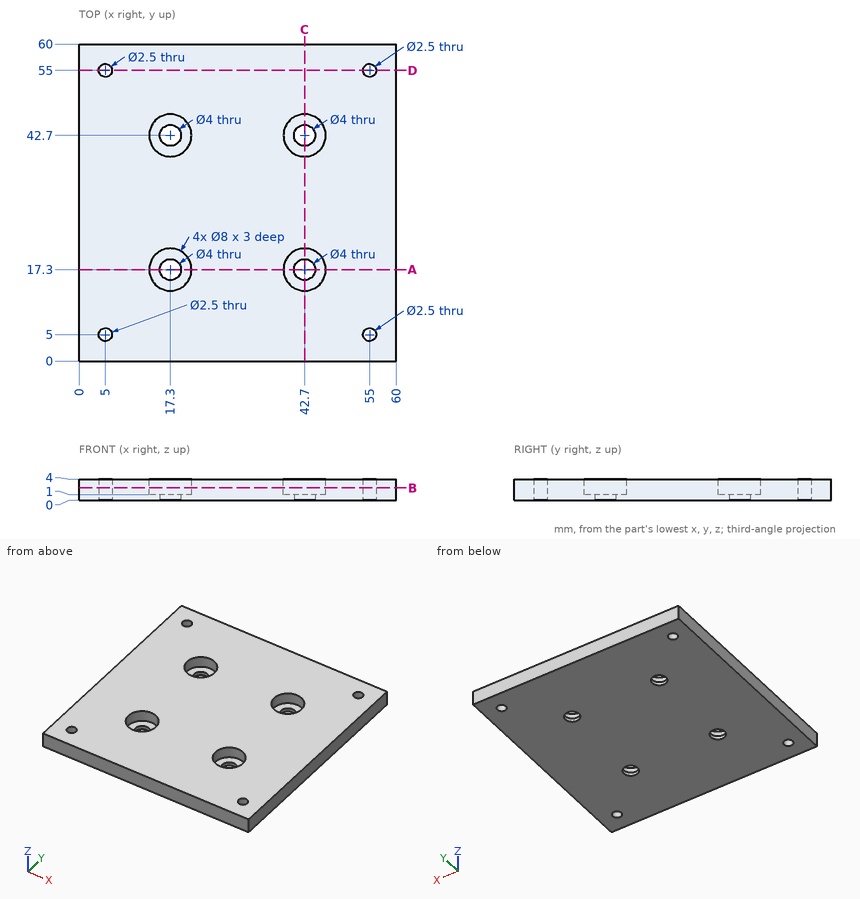
Geometry: see drawing. Coordinates: mm, zero at the bounding-box minimum. Coordinates: 2 decimals unless noted, no trailing zeros. Order: outer loops, then holes, each group sorted by start corner. A loop starts at its lowest first (then second) coordinate and runs counter-clockwise, first axis right, second up. Notation, with made-up numbers: M 59.25,-26 L 98.25,-26 A14 ccw 98.25,-3 Z; hole C 23.5,57 d2. An arc over 180 degrees is marked long. Write each question's results on one line, items separated by ' | '. Start each with the question number.
1) Section query D-D (y = 55). Return the cut outline in (x, z).
2) Section query A-A (y = 17.3). Return the cut outline in (x, z).
3) Section query B-B (z = 2.3). Give the number of separate pieces and of enclosed holes in the cut face, plus the area to 3 significant figures.
4) Contact query for flat-ended pins moving along their axis: pin 1 Ø13 at (x, y) = (17.3, 42.7) entering from -Z; pin 2 Ø2.5 at (x, y) = (17.3, 17.3) entering from +Z; pin 3 Ø4 at (x, y) = (44, 43) entering from +Z. Output: stop coordinate, or through.
5) Line query: line 1 (Y direction, x = 55, z = 2.35); line 2 (Y direction, x = 17.3, z = 0.3); line 3 (X direction, y = 17.5, z = 0.2). Output: solid intervals per line, ascending. Write a range as from..to.
Answers:
1) outline: M 0,0 L 3.75,0 L 3.75,4 L 0,4 Z; M 6.25,0 L 53.75,0 L 53.75,4 L 6.25,4 Z; M 56.25,0 L 60,0 L 60,4 L 56.25,4 Z
2) outline: M 0,0 L 15.3,0 L 15.3,1 L 13.3,1 L 13.3,4 L 0,4 Z; M 19.3,0 L 40.7,0 L 40.7,1 L 38.7,1 L 38.7,4 L 21.3,4 L 21.3,1 L 19.3,1 Z; M 44.7,0 L 60,0 L 60,4 L 46.7,4 L 46.7,1 L 44.7,1 Z
3) separate pieces: 1 | enclosed holes: 8 | area: 3,380 mm^2
4) pin 1: stops at z = 0 | pin 2: passes through | pin 3: stops at z = 1
5) line 1: y = 0..3.75, 6.25..53.75, 56.25..60 | line 2: y = 0..15.3, 19.3..40.7, 44.7..60 | line 3: x = 0..15.31, 19.29..40.71, 44.69..60
